Drawing for the job (mm, zero at the part's lowest x, y, z). Give positions to 0.01 mm unless a question says otherwise; leave off trailing zeros. Order: outer loops, then holes, each group sorted by start corner. A loop starts at its lowest first (then second) coordinate and runs counter-clockwise, first axis right, second up. Notation, with made-up numbers: (15, 43) - (53, 43) arc R23 cw to (53, 75) - close; hole circle Ø8 at (13.5, 29). An arc over 180 degrees is marked (long way). Use a Markdown table: item, result.
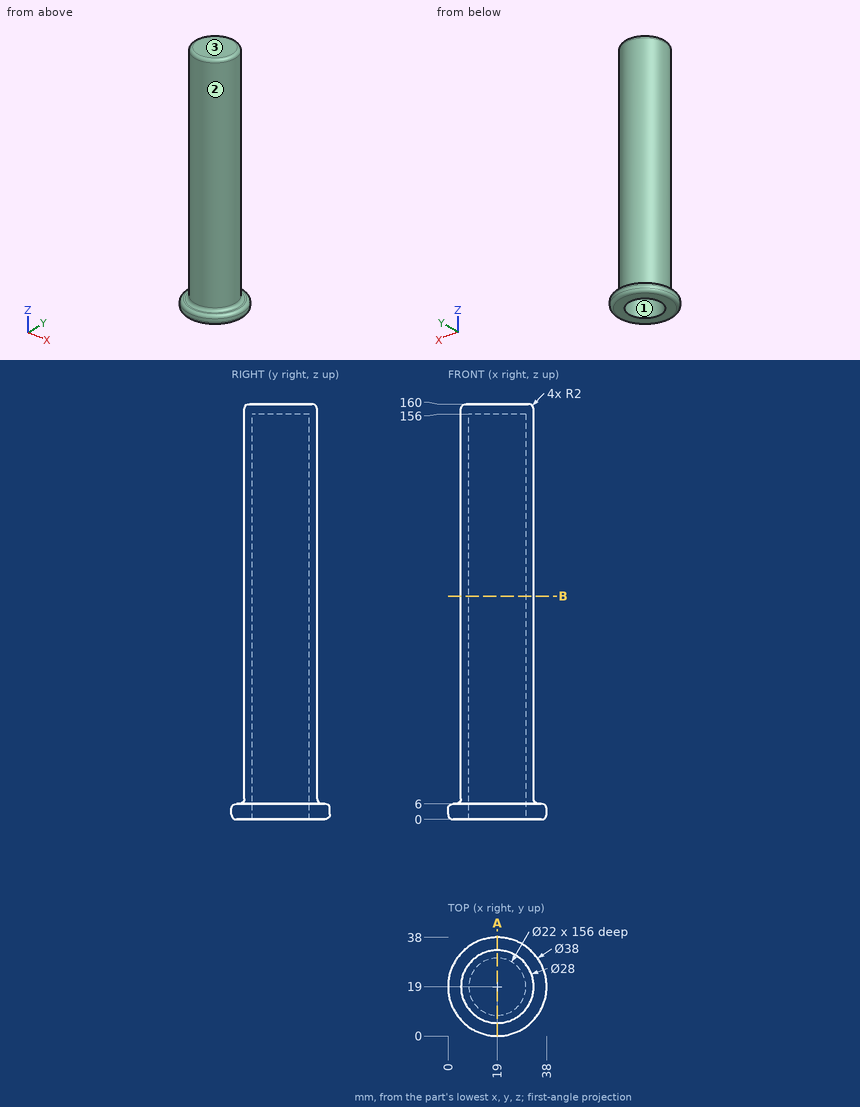
1) Slice it at A-A (x = 19). Write the cut outline in (y, z), and give its area (3 significant figures).
Computed:
| item | result |
|---|---|
| outline | (0, 2) arc R2 ccw to (2, 0) - (8, 0) - (8, 156) - (30, 156) - (30, 0) - (36, 0) arc R2 ccw to (38, 2) - (38, 4) arc R2 ccw to (36, 6) - (35, 6) arc R2 cw to (33, 8) - (33, 158) arc R2 ccw to (31, 160) - (7, 160) arc R2 ccw to (5, 158) - (5, 8) arc R2 cw to (3, 6) - (2, 6) arc R2 ccw to (0, 4) - close |
| area | 1,100 mm² |
2) Slice it at B-B (z = 86). Write the cut outline in (x, y), and give its area (3 significant figures).
Computed:
| item | result |
|---|---|
| outline | circle Ø28 at (19, 19); hole circle Ø22 at (19, 19) |
| area | 236 mm² |
3) Wall check: line 1 (Y direction, x = 19, z = 46); line 2 (Z direction, x = 11, y = 4.5); line 3 (Z direction, x = 23, y = 22). Give the ranges that are in metal, low to high. Write a range as from..to.
Computed:
| item | result |
|---|---|
| line 1 | y = 5..8, 30..33 |
| line 2 | z = 0..6 |
| line 3 | z = 156..160 |
4) Two-plate mould, pull along X, no slides. Class the marked faces 1, 2 and 3: +X half, -X half, draft (parallel to the pull), parting line (faces both ways), or undercut.
Computed:
| item | result |
|---|---|
| face 1 | undercut |
| face 2 | parting line |
| face 3 | draft |
5) Pin check, flat tips, straight feed: P1, Ø10, axis at y = 19.5, z = 22, coming from the +X side; P2, Ø2, axis at x = 19, z = 56.5, coming from the +Y side; P3, Ø12, axis at y = 9, z = 37, coming from the -X side. Stop position of each tip, or through.
Computed:
| item | result |
|---|---|
| P1 | stops at x = 33 |
| P2 | stops at y = 33 |
| P3 | stops at x = 5.58 |
